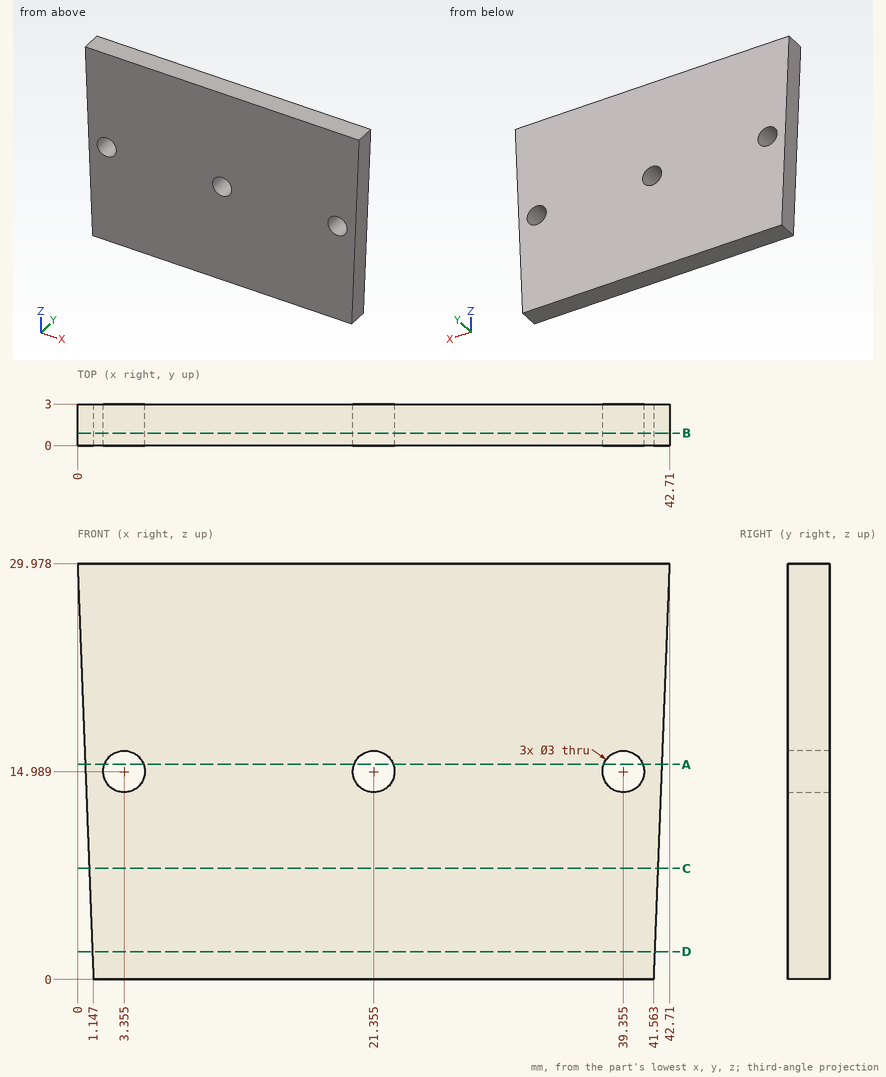
Geometry check sheet. Reference: drawing and pictorial views, mm from the part's lowest x, y, z. Coordinates: 2 decimals unless noted, no trailing zeros. Write each loop counter-clockwise with the first axis right and the second up, starting at its lowest first coordinate (ties: lowest second). Pieces come first, ordered by that corner, then holes. Notation, with made-up numbers: M -17,-13 L 35,-13 A15 ccw 35,-4 Z; hole C 10.5,39 d3. An arc over 180 degrees is marked long. One line per question, with ' | ' between items.
1) Sectioned sample at D-D on z = 2. Record the cut outline in (x, y), then the cut area to 3 significant figures.
Solutions:
outline: M 1.07,0 L 41.64,0 L 41.64,3 L 1.07,3 Z | area: 122 mm^2
2) Sectioned sample at C-C on z = 8. Record the cut outline in (x, y), then the cut area to 3 significant figures.
Solutions:
outline: M 0.84,0 L 41.87,0 L 41.87,3 L 0.84,3 Z | area: 123 mm^2
3) Sectioned sample at A-A on z = 15.5. Record the cut outline in (x, y), then the cut area to 3 significant figures.
Solutions:
outline: M 0.55,0 L 1.94,0 L 1.94,3 L 0.55,3 Z; M 4.77,0 L 19.94,0 L 19.94,3 L 4.77,3 Z; M 22.77,0 L 37.94,0 L 37.94,3 L 22.77,3 Z; M 40.77,0 L 42.16,0 L 42.16,3 L 40.77,3 Z | area: 99.4 mm^2
4) Sectioned sample at B-B on y = 0.9. Record the cut outline in (x, z) (3 decimals), then the cut area to 3 significant figures.
Solutions:
outline: M 0,29.978 L 1.147,0 L 41.563,0 L 42.71,29.978 Z; hole C 3.355,14.989 d3; hole C 21.355,14.989 d3; hole C 39.355,14.989 d3 | area: 1,220 mm^2
5) Material ranges on L1, parallel to X at y = 1.1, z = 14.25; L2, parallel to Z at x = 4.5, y = 2; L3, parallel to Z at x = 3, y = 0.65, recorded low to high.
Solutions:
L1: 0.6 to 2.05, 4.66 to 20.05, 22.66 to 38.05, 40.66 to 42.11 | L2: 0 to 14.02, 15.96 to 29.98 | L3: 0 to 13.53, 16.45 to 29.98
